```python
from build123d import *

# Parameters (mm, degrees)
SKETCH_1_R          = 30
SKETCH_1_R_2        = 11.5
EXTRUDE_1_DEPTH     = 30
SKETCH_1_3_R        = 11.5
EXTRUDE_2_DEPTH     = 70
EXTRUDE_3_DEPTH     = 10
FILLET_1_RADIUS     = 5
FILLET_1_LENGTH     = 10
FILLET_2_RADIUS     = 5
FILLET_2_LENGTH     = 10
SKETCH_4_R          = 1.5
CUT_EXTRUDE_1_DEPTH = 78.888432891
FILLET_3_R          = 2


with BuildPart() as part:
    # 草圖1 → 填料-伸長1 (new body)
    # profile 1 of 2: a face of its own
    with BuildSketch(Plane(origin=(0, 0, 0), x_dir=(1, 0, 0), z_dir=(0, 1, 0))):
        with Locations(Location((0, 0, 0), (0, 0, 270))):
            Circle(SKETCH_1_R)
        Circle(SKETCH_1_R_2, mode=Mode.SUBTRACT)
    # profile 2 of 2: a face of its own
    with BuildSketch(Plane(origin=(0, 0, 0), x_dir=(1, 0, 0), z_dir=(0, 1, 0))):
        Circle(SKETCH_1_R_2)
    extrude(amount=EXTRUDE_1_DEPTH)

    # 草圖1<3> → 填料-伸長2 (add)
    with BuildSketch(Plane(origin=(0, 0, 0), x_dir=(1, 0, 0), z_dir=(0, 1, 0))):
        with Locations(Location((0, 0, 0), (0, 0, 270))):
            Circle(SKETCH_1_3_R)
    extrude(amount=EXTRUDE_2_DEPTH)

    # 草圖3 → 填料-伸長3 (add)
    with BuildSketch(Plane.XZ):
        with BuildLine():
            Line((29.580398915, 5), (39.580398915, 5))
            Line((39.580398915, 5), (39.580398915, -5))
            Line((39.580398915, -5), (29.580398915, -5))
            ThreePointArc((29.580398915, -5), (30, 0), (29.580398915, 5))
        make_face()
        with BuildLine():
            Line((-29.580398915, -5), (-39.580398915, -5))
            Line((-39.580398915, -5), (-39.580398915, 5))
            Line((-39.580398915, 5), (-29.580398915, 5))
            ThreePointArc((-29.580398915, 5), (-30, 0), (-29.580398915, -5))
        make_face()
    extrude(amount=-EXTRUDE_3_DEPTH)

    # 圓角1: full round fillet: the end face becomes a half cylinder, R = half its width
    fillet_1_face = Plane((-39.580398915, 5, 0), x_dir=(0, -1, 0), z_dir=(-1, 0, 0))  # on the end face: x along it, z out of the body
    fillet_1_slab = fillet_1_face.offset(-FILLET_1_RADIUS / 2) * Box(FILLET_1_LENGTH, 2 * FILLET_1_RADIUS, FILLET_1_RADIUS, mode=Mode.PRIVATE)  # the body's end, R deep
    fillet_1_round = Plane((-34.580398915, 5, 0), x_dir=(-1, 0, 0), z_dir=(0, -1, 0)) * Cylinder(FILLET_1_RADIUS, FILLET_1_LENGTH, mode=Mode.PRIVATE)  # its axis R under the face
    add(fillet_1_slab - fillet_1_round, mode=Mode.SUBTRACT)

    # 圓角2: full round fillet: the end face becomes a half cylinder, R = half its width
    fillet_2_face = Plane((39.580398915, 5, 0), x_dir=(0, 1, 0), z_dir=(1, 0, 0))  # on the end face: x along it, z out of the body
    fillet_2_slab = fillet_2_face.offset(-FILLET_2_RADIUS / 2) * Box(FILLET_2_LENGTH, 2 * FILLET_2_RADIUS, FILLET_2_RADIUS, mode=Mode.PRIVATE)  # the body's end, R deep
    fillet_2_round = Plane((34.580398915, 5, 0), x_dir=(1, 0, 0), z_dir=(0, 1, 0)) * Cylinder(FILLET_2_RADIUS, FILLET_2_LENGTH, mode=Mode.PRIVATE)  # its axis R under the face
    add(fillet_2_slab - fillet_2_round, mode=Mode.SUBTRACT)

    # 草圖4 → 除料-伸長1 (cut, through all)
    with BuildSketch(Plane(origin=(0, 10, 0), x_dir=(1, 0, 0), z_dir=(0, 1, 0))):
        with Locations(Location((34.580398915, 0, 0), (0, 0, 270))):
            Circle(SKETCH_4_R)
        with Locations(Location((-34.580398915, 0, 0), (0, 0, 270))):
            Circle(SKETCH_4_R)
    extrude(amount=-CUT_EXTRUDE_1_DEPTH, mode=Mode.SUBTRACT)

    # 圓角3
    fillet_3_edges = [part.edges().sort_by_distance(p)[0] for p in [
        (0, 30, -30),
        (0, 70, -11.5),
    ]]
    fillet(fillet_3_edges, radius=FILLET_3_R)


solid = part.part
```
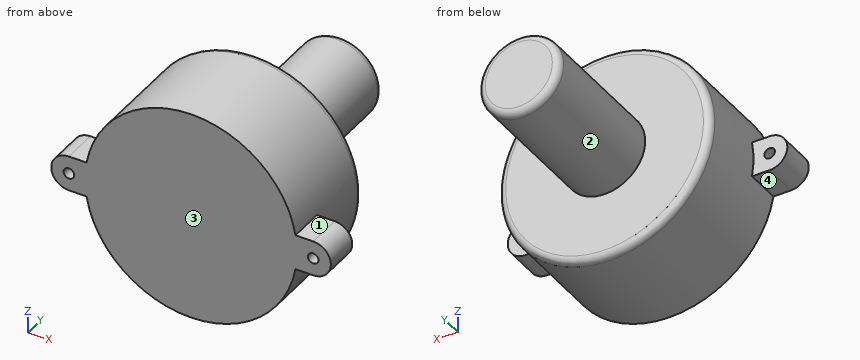
CAD build for the part. Positions are in the model's coordinates, mm. Face numbers are marked on the shaded views. A direction names the side the tool comes from. Round coordinates to 2 decimals unless told otherwise and drop trailing zeros. Loops run counter-clockwise (first coordinate to the right, second up) from the corner with the lowest first, then second, coordinate; pieces in that order, holes last. Notation, with made-up numbers: M 10.25,-1 L 55.25,-1 A18 cw 55.25,5 Z; hole C 80.5,25.25 d7. An arc over 180 degrees is marked long. Use a Markdown table: item, result. Add a question column.
(1) Cut at D-D (x = 31.5). Give the cut face in (y, z), and give its area (3 significant figures).
(2) Drill centre lines: line 1 (X direction, y = 3.25, z = 0); line 2 (Y direction, x = -21, z = 6.5); line 3 (X direction, y = 35.5, z = 8). Where is each one in solid material? Low to high.
(3) Which spindle directions (+Z, -Z, +X, -X, +Y, -Y) get a long thin tool onto all of the face, cutting with end or side? Do the marked faces 1, 2, 3 and 4. Say none if no direction does.
(4) Cut at A-A (z = 0). Give the cut face in (x, y), and give its area (3 significant figures).
(5) Cut at B-B (x = 0). Give the cut face in (y, z).
(6) Cut at C-C (y = 26.5). Give the cut face in (x, z), and give its area (3 significant figures).
(7) Flat gauge pins, fed straight in: pin 1 (11 mm diameter, centred on x = -35, z = 0, fed in from +Y); pin 2 (5 mm diameter, centred on x = 2.5, z = 9.5, fed in from -Y); pin 3 (2.5 mm diameter, centred on x = 33, y = 3, fed in from -Z); pin 4 (3.5 mm diameter, centred on x = 34.58, z = 0, fed in from +Y). Where does each tip first touch, or does it go through?
Geometry says:
| question | item | result |
|---|---|---|
| 1 | outline | M 0,-5 L 10,-5 L 10,5 L 0,5 Z |
| 1 | area | 100 mm² |
| 2 | line 1 | x = -39.58 to -36.08, -33.08 to 33.08, 36.08 to 39.58 |
| 2 | line 2 | y = 0 to 30 |
| 2 | line 3 | x = -8.26 to 8.26 |
| 3 | face 1 | +Z, +X, +Y, -Y |
| 3 | face 2 | +Y |
| 3 | face 3 | +Z, -Z, +X, -X, -Y |
| 3 | face 4 | -Z, -X, +Y, -Y |
| 4 | outline | M -39.58,0 L -36.08,0 L -36.08,10 L -39.58,10 Z; M -33.08,0 L 33.08,0 L 33.08,10 L 30,10 L 30,28 A2 ccw 28,30 L 11.5,30 L 11.5,68 A2 ccw 9.5,70 L -9.5,70 A2 ccw -11.5,68 L -11.5,30 L -28,30 A2 ccw -30,28 L -30,10 L -33.08,10 Z; M 36.08,0 L 39.58,0 L 39.58,10 L 36.08,10 Z |
| 4 | area | 2,850 mm² |
| 5 | outline | M 0,-30 L 28,-30 A2 ccw 30,-28 L 30,-11.5 L 68,-11.5 A2 ccw 70,-9.5 L 70,9.5 A2 ccw 68,11.5 L 30,11.5 L 30,28 A2 ccw 28,30 L 0,30 Z |
| 6 | outline | C 0,0 d60 |
| 6 | area | 2,830 mm² |
| 7 | pin 1 | stops at y = 29.32 |
| 7 | pin 2 | stops at y = 0 |
| 7 | pin 3 | stops at z = -5 |
| 7 | pin 4 | stops at y = 10 |
